Geometry: final body of the model. Coordinates: model frame, mm. A direction names the side the tool comes from. Round coordinates to 2 decimals unless told otherwise and drop trailing zeros. Loops run counter-clockwise (first coordinate to the right, second up) from the corner with the lowest first, then second, coordinate; pieces in that order, holes last. Notation, with made-up numbers: (47.5, -25.75) -> (53.5, -25.75) arc R11 ccw to (53.5, -16.75) -> close; hole circle Ø11 at (79.25, 28). An arc over 180 degrees is marked (long way). Answer in a Markdown table with one row per item.
```python
from build123d import *

# Parameters (mm, degrees)
SKETCH_1_R                   = 27.5
SKETCH_1_R_2                 = 21
EXTRUDE_1_DEPTH              = 6
SKETCH_1_3_R                 = 21
SKETCH_1_3_R_2               = 19.61
EXTRUDE_2_DEPTH              = 1.5
HOLE_WIZARD_M3_1_D           = 3.2
HOLE_WIZARD_M3_1_CSINK_D     = 6.3
HOLE_WIZARD_M3_1_CSINK_ANGLE = 90


with BuildPart() as part:
    # ｽｹｯﾁ1 → ﾎﾞｽ - 押し出し1 (new body)
    with BuildSketch(Plane.XY):
        Circle(SKETCH_1_R)
        Circle(SKETCH_1_R_2, mode=Mode.SUBTRACT)
    extrude(amount=EXTRUDE_1_DEPTH)

    # ｽｹｯﾁ1<3> → ﾎﾞｽ - 押し出し2 (add)
    with BuildSketch(Plane.XY):
        Circle(SKETCH_1_3_R)
        Circle(SKETCH_1_3_R_2, mode=Mode.SUBTRACT)
    extrude(amount=EXTRUDE_2_DEPTH)

    # M3 丸皿ねじ用皿穴1 (through all)
    with Locations(Plane(origin=(16.970562748, 16.970562748, 0), x_dir=(-1, 0, 0), z_dir=(0, 0, -1))):
        with Locations((0, 0), (33.941125496, 0), (33.941125496, -33.941125496), (0, -33.941125496)):
            CounterSinkHole(HOLE_WIZARD_M3_1_D / 2, HOLE_WIZARD_M3_1_CSINK_D / 2, counter_sink_angle=HOLE_WIZARD_M3_1_CSINK_ANGLE)


solid = part.part
```
Item 1: Section query D-D, the plane x = 24. Output: boundary loops of the cut face in (y, z), and give its area (3 significant figures).
Ans:
| item | result |
|---|---|
| outline | (-13.43, 0) -> (13.43, 0) -> (13.43, 6) -> (-13.43, 6) -> close |
| area | 161 mm2 |
Item 2: Ray query, L1, parallel to Y at x = 0, z = 4.7; L2, parallel to Z at x = -19, y = -7; L3, parallel to Y at x = -15, z = 0.9. Return the intervals inside material, ascending.
Ans:
| item | result |
|---|---|
| L1 | -27.5 to -21, 21 to 27.5 |
| L2 | 0 to 1.5 |
| L3 | -23.05 to -18.06, -15.88 to -12.63, 12.63 to 15.88, 18.06 to 23.05 |
Item 3: Section query A-A, the plane x = 0. Output: boundary loops of the cut face in (y, z), and give its area (3 significant figures).
Ans:
| item | result |
|---|---|
| outline | (-27.5, 0) -> (-19.61, 0) -> (-19.61, 1.5) -> (-21, 1.5) -> (-21, 6) -> (-27.5, 6) -> close; (19.61, 0) -> (27.5, 0) -> (27.5, 6) -> (21, 6) -> (21, 1.5) -> (19.61, 1.5) -> close |
| area | 82.2 mm2 |
Item 4: First-contact query: P1, Ø1, axis at y = 1, z = 4.5, coming from the -X side; P2, Ø4, axis at x = 16.97, y = -16.97, coming from the -Z side; P3, Ø1.5, axis at x = -6, z = 5, coming from the -Y side. Flat tips, straight axial feed; report the tip coordinate or a pass-through.
Ans:
| item | result |
|---|---|
| P1 | x = -27.5 |
| P2 | z = 1.15 |
| P3 | y = -26.99 |
Item 5: Section query B-B, the plane y = 6.5. Output: boundary loops of the cut face in (x, z), and give its area (3 significant figures).
Ans:
| item | result |
|---|---|
| outline | (-26.72, 0) -> (-18.5, 0) -> (-18.5, 1.5) -> (-19.97, 1.5) -> (-19.97, 6) -> (-26.72, 6) -> close; (18.5, 0) -> (26.72, 0) -> (26.72, 6) -> (19.97, 6) -> (19.97, 1.5) -> (18.5, 1.5) -> close |
| area | 85.4 mm2 |
Item 6: Section query C-C, the plane z = 2.95. Output: boundary loops of the cut face in (x, y).
Ans:
| item | result |
|---|---|
| outline | circle Ø55 at (0, 0); hole circle Ø42 at (0, 0); hole circle Ø3.2 at (-16.97, -16.97); hole circle Ø3.2 at (-16.97, 16.97); hole circle Ø3.2 at (16.97, -16.97); hole circle Ø3.2 at (16.97, 16.97) |
Item 7: Set-up query: faces 4 (the cylindrical face through (20.03, 6.31, 3.72)), 5 (the cylindrical face through (-18.24, -17.944, 3.806)). Return all of +Z, -Z, +X, -X, +Y, -Y with unobstructed straight access to the full face (end or side cutting, diameter ignored); none if empty.
Ans:
| item | result |
|---|---|
| face 4 | +Z |
| face 5 | +Z, -Z |
Item 8: Mould query, pull axis Y, two halves, no side actions, for faces 1 (the flat face through (14, -14, 0)), 2 (the cylindrical face through (-5.961, -26.846, 2.958)), 3 (the cylindrical face through (-17.32, 15.41, 3.81)). Classes: released by +Y, released by -Y, zero draft, split by the parting line, or undercut.
Ans:
| item | result |
|---|---|
| face 1 | zero draft |
| face 2 | split by the parting line |
| face 3 | undercut |
